Design review of the part built by this model. Coordinates are the model's own, in mm. Face numbers are marked on the shaded views. A direction names the side the tool comes from. Give positions to 0.01 mm unless a question says otherwise; leave off trailing zeros. Write each loop counter-clockwise with the first axis right and the second up, starting at its lowest first coordinate (ties: lowest second). Pieces come first, ordered by that corner, then holes.
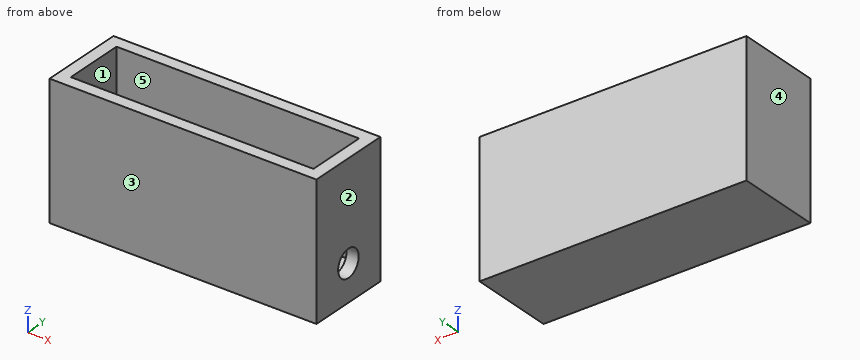
```python
from build123d import *

# Parameters (mm, degrees)
ESBO_O1_W                = 44
ESBO_O1_H                = 14
RESSALTO_EXTRUS_O1_DEPTH = 22
ESBO_O2_W                = 40
ESBO_O2_H                = 10
CORTE_EXTRUS_O1_DEPTH    = 19
ESBO_O3_R                = 2.25
CORTE_EXTRUS_O2_DEPTH    = 5


with BuildPart() as part:
    # Esboço1 → Ressalto-extrusão1 (new body)
    with BuildSketch(Plane.XY):
        Rectangle(ESBO_O1_W, ESBO_O1_H)
    extrude(amount=RESSALTO_EXTRUS_O1_DEPTH)

    # Esboço2 → Corte-extrusão1 (cut)
    with BuildSketch(Plane.XY.offset(22)):
        Rectangle(ESBO_O2_W, ESBO_O2_H)
    extrude(amount=-CORTE_EXTRUS_O1_DEPTH, mode=Mode.SUBTRACT)

    # Esboço3 → Corte-extrusão2 (cut)
    with BuildSketch(Plane(origin=(22, 0, 0), x_dir=(0, 0, -1), z_dir=(1, 0, 0))):
        with Locations((-6, 0)):
            Circle(ESBO_O3_R)
    extrude(amount=-CORTE_EXTRUS_O2_DEPTH, mode=Mode.SUBTRACT)


solid = part.part
```
(1) Consider section B-B, the plane y = 0. Give the boundary of the cut face in (x, z).
Resolved:
outline: (-22, 0) - (22, 0) - (22, 3.75) - (20, 3.75) - (20, 3) - (-20, 3) - (-20, 22) - (-22, 22) - close; (20, 8.25) - (22, 8.25) - (22, 22) - (20, 22) - close
(2) Consider section D-D, the plane z = 6. Give the boundary of the cut face in (x, y).
Resolved:
outline: (-22, -7) - (22, -7) - (22, -2.25) - (20, -2.25) - (20, -5) - (-20, -5) - (-20, 5) - (20, 5) - (20, 2.25) - (22, 2.25) - (22, 7) - (-22, 7) - close
(3) Tool access review of the marked faces 1 and 2: name each direction out of +Z, -Z, +X, -X, +Y, -Y from which nothing blocks a thin tool from reaching the whole face with its end or side.
Resolved:
face 1: +Z
face 2: +Z, -Z, +X, +Y, -Y
(4) Clearance check with flat-ended pins moving along their axes: P1, Ø4, axis at y = 0, z = 6, coming from the +X side; P2, Ø3, axis at x = -11, y = 3, coming from the +Z side. State where each tip first meets the part, or that it passes through.
Resolved:
P1: stops at x = -20
P2: stops at z = 3
(5) Consider section C-C, the plane x = -15.5. Give the boundary of the cut face in (y, z), then the cut area to 3 significant figures.
Resolved:
outline: (-7, 0) - (7, 0) - (7, 22) - (5, 22) - (5, 3) - (-5, 3) - (-5, 22) - (-7, 22) - close
area: 118 mm2
(6) To check wall thickness, follow L1, parallel to Y at x = 4, z = 3.75; L2, parallel to Y at x = 21.2, z = 6; L3, parallel to X at y = 3.5, z = 18. State the ranges of each line that lie inside material, in increasing order.
Resolved:
L1: y = -7 to -5, 5 to 7
L2: y = -7 to -2.25, 2.25 to 7
L3: x = -22 to -20, 20 to 22
(7) Consider section A-A, the plane z = 11. Give the boundary of the cut face in (x, y), then the cut area to 3 significant figures.
Resolved:
outline: (-22, -7) - (22, -7) - (22, 7) - (-22, 7) - close; hole (-20, -5) - (20, -5) - (20, 5) - (-20, 5) - close
area: 216 mm2
(8) Mouldability with a two-part tool opening along Y and no side actions: class the marked faces 3, 4 and 5 as pulls with the +Y half, pulls with the -Y half, needs draft (parallel to the pull), parting line crosses it, or undercut.
Resolved:
face 3: pulls with the -Y half
face 4: needs draft
face 5: undercut
